Geometry: see drawing. Coordinates: mm, zero at the bounding-box minimum. A direction names the side the tool comes from. Coordinates: 2 decimals unless noted, no trailing zeros. Loops run counter-clockwise (first coordinate to the right, second up) from the corner with the lowest first, then second, coordinate; pieces in that order, holes last. Notation, with made-up numbers: (-36.75, 55.25) - (15.25, 55.25) arc R15 ccw to (15.25, 63.25) - close; hole circle Ø2 at (27.25, -35.5). An arc over 180 degrees is marked (long way). Use a Markdown table: item, result. Add a question column.
1. Section query B-B on z = 18.5. Return the cut outline in (x, y), then the cut area to 3 significant figures.
2. Section query C-C on z = 10. Return the cut outline in (x, y).
3. Contact query for flat-ended pins moving along their axis: P1, Ø12, axis at x = 46, z = 11.5, coming from the +Y side; P2, Ø8, axis at x = 35.5, y = 14.5, coming from the -Z side. Output: stop coordinate, or through.
4. Section query D-D on y = 47.5. Return the cut outline in (x, z), then the cut area to 3 significant figures.
5. Ray query, L1, parallel to Y at x = 0.9, z = 8.5; L2, parallel to X at y = 41.5, z = 11; L3, parallel to Z at x = 4, y = 28. Return the intervals inside material, ascending. Write a range as [from, to].
6. Section query A-A on y = 15. Return the cut outline in (x, z).
7. Draft query along Z for the marked faces 1, 2 and 3. Return one class per face: released by +Z, released by -Z, zero draft, split by the parting line, or undercut.
8. Access query for the marked faces 4 and 5. Directions: +Z, -Z, +X, -X, +Y, -Y. A direction counts if a zero-diameter tool reaches every point of the face in a straight line with its end or side. Return the directions, or none.
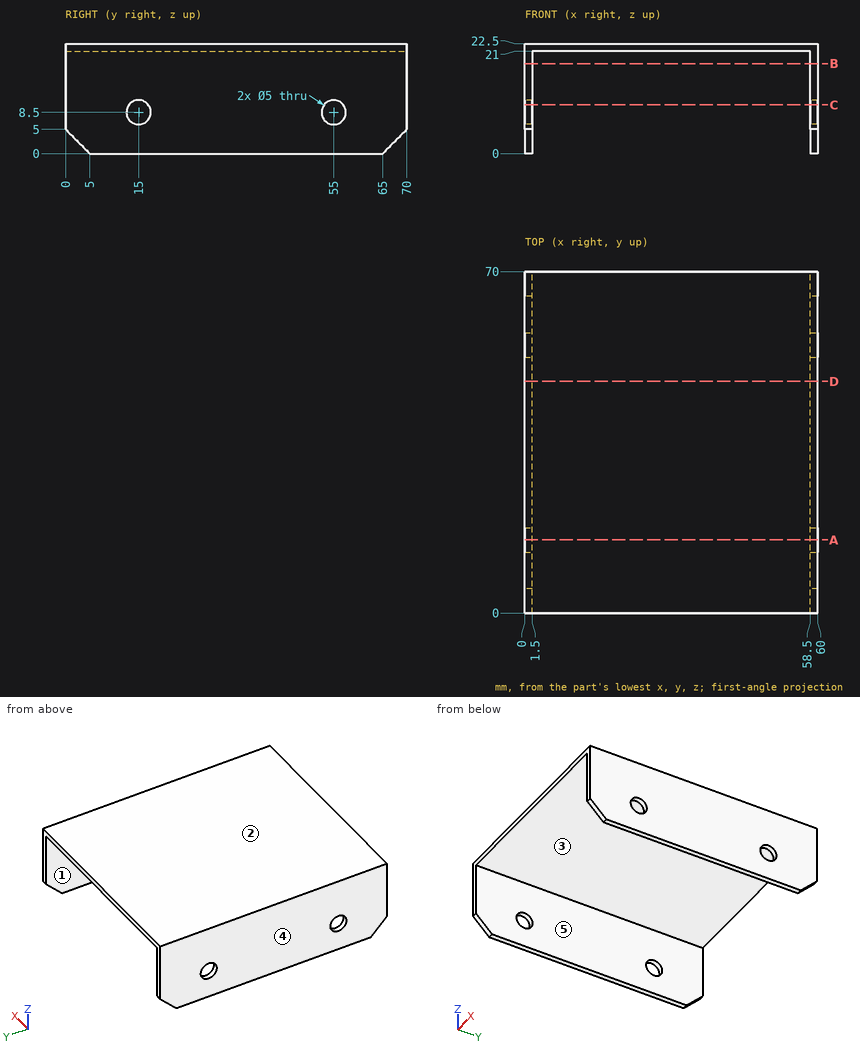
Resolved:
| question | item | result |
|---|---|---|
| 1 | outline | (0, 0) - (1.5, 0) - (1.5, 70) - (0, 70) - close; (58.5, 0) - (60, 0) - (60, 70) - (58.5, 70) - close |
| 1 | area | 210 mm² |
| 2 | outline | (0, 0) - (1.5, 0) - (1.5, 13) - (0, 13) - close; (0, 17) - (1.5, 17) - (1.5, 53) - (0, 53) - close; (0, 57) - (1.5, 57) - (1.5, 70) - (0, 70) - close; (58.5, 0) - (60, 0) - (60, 13) - (58.5, 13) - close; (58.5, 17) - (60, 17) - (60, 53) - (58.5, 53) - close; (58.5, 57) - (60, 57) - (60, 70) - (58.5, 70) - close |
| 3 | P1 | through |
| 3 | P2 | z = 21 |
| 4 | outline | (0, 0) - (1.5, 0) - (1.5, 21) - (58.5, 21) - (58.5, 0) - (60, 0) - (60, 22.5) - (0, 22.5) - close |
| 4 | area | 153 mm² |
| 5 | L1 | [0, 12.5], [17.5, 52.5], [57.5, 70] |
| 5 | L2 | [0, 1.5], [58.5, 60] |
| 5 | L3 | [21, 22.5] |
| 6 | outline | (0, 0) - (1.5, 0) - (1.5, 6) - (0, 6) - close; (0, 11) - (1.5, 11) - (1.5, 21) - (58.5, 21) - (58.5, 11) - (60, 11) - (60, 22.5) - (0, 22.5) - close; (58.5, 0) - (60, 0) - (60, 6) - (58.5, 6) - close |
| 7 | face 1 | zero draft |
| 7 | face 2 | released by +Z |
| 7 | face 3 | released by -Z |
| 8 | face 4 | +Z, -Z, -X, +Y, -Y |
| 8 | face 5 | -Z, +Y, -Y |
